from build123d import *

# Parameters (mm, degrees)
SKETCH2_R              = 26
BOSS_EXTRUDE2_DEPTH    = 5
SKETCH3_R              = 4
CUT_EXTRUDE1_DEPTH     = 2
CUT_EXTRUDE3_START     = -5
CUT_EXTRUDE3_OUTLINE_R = 26
CUT_EXTRUDE3_DEPTH     = 5


# Read off the part's stored shape, not the designer's step: Cut-Extrude3
with BuildPart() as part:
    # Sketch2 → Boss-Extrude2 (new body)
    with BuildSketch(Plane(origin=(0, 0, 0), x_dir=(1, 0, 0), z_dir=(0, 1, 0))):
        with Locations(Location((0, 0, 0), (0, 0, 270))):
            Circle(SKETCH2_R)
    extrude(amount=BOSS_EXTRUDE2_DEPTH)

    # Sketch3 → Cut-Extrude1 (cut)
    with BuildSketch(Plane.XZ.offset(-5)):
        with Locations(Location((9.52625, -16.499949006, 0), (0, 0, 270))):
            Circle(SKETCH3_R)
        with Locations(Location((9.52625, 16.499949006, 0), (0, 0, 270))):
            Circle(SKETCH3_R)
        with Locations(Location((-19.0525, 0, 0), (0, 0, 270))):
            Circle(SKETCH3_R)
    extrude(amount=CUT_EXTRUDE1_DEPTH, mode=Mode.SUBTRACT)

    # Cut-Extrude3 outline → Cut-Extrude3 (cut)
    # profile 1 of 2: a face of its own
    with BuildSketch(Plane(origin=(0, 5, 0), x_dir=(1, 0, 0), z_dir=(0, 1, 0)).offset(CUT_EXTRUDE3_START)):
        Circle(CUT_EXTRUDE3_OUTLINE_R)
        with BuildLine():
            ThreePointArc((-19.664092803, -5.96874813), (-25.0525, 0), (-19.664092803, 5.96874813))
            ThreePointArc((-19.664092803, 5.96874813), (-10.275, 17.796822048), (4.662958892, 20.013977975))
            ThreePointArc((4.662958892, 20.013977975), (12.52625, 21.696101428), (15.001133911, 14.045229844))
            ThreePointArc((15.001133911, 14.045229844), (20.55, 0), (15.001133911, -14.045229844))
            ThreePointArc((15.001133911, -14.045229844), (12.52625, -21.696101428), (4.662958892, -20.013977975))
            ThreePointArc((4.662958892, -20.013977975), (-10.275, -17.796822048), (-19.664092803, -5.96874813))
        make_face(mode=Mode.SUBTRACT)
    # profile 2 of 2: a face of its own
    with BuildSketch(Plane(origin=(0, 5, 0), x_dir=(1, 0, 0), z_dir=(0, 1, 0)).offset(CUT_EXTRUDE3_START)):
        with BuildLine():
            ThreePointArc((-16.664486452, 5.504306613), (-13.0525, 0), (-16.664486452, -5.504306613))
            ThreePointArc((-16.664486452, -5.504306613), (-8.775, -15.198745836), (3.565373869, -17.184021915))
            ThreePointArc((3.565373869, -17.184021915), (6.52625, -11.303796583), (13.099112583, -11.679715302))
            ThreePointArc((13.099112583, -11.679715302), (17.55, 0), (13.099112583, 11.679715302))
            ThreePointArc((13.099112583, 11.679715302), (6.52625, 11.303796583), (3.565373869, 17.184021915))
            ThreePointArc((3.565373869, 17.184021915), (-8.775, 15.198745836), (-16.664486452, 5.504306613))
        make_face()
    extrude(amount=CUT_EXTRUDE3_DEPTH, mode=Mode.SUBTRACT)


solid = part.part
Check sheet for the modelled part. Datum: model origin and axes. Units: mm. A direction names the side the tool comes from. Give positions to 0.01 mm unless a question says otherwise; leave off trailing zeros. Loops run counter-clockwise (first coordinate to the right, second up) from the corner with the lowest first, then second, coordinate; pieces in that order, holes last. Notation, with made-up numbers: M -13.75,-5 L -2.75,-5 A16 ccw -2.75,6 Z; hole C 76.5,-1.5 d6. An arc over 180 degrees is marked long. Answer as a JSON object with one key per item and string values. Group by question number.
Q1. Access from +Z, -Z, +X, -X, +Y, -Y to the whole of each face (thin tool, end or side, straight path). Record for faces 4 (the cylindrical face through (6.611, 2.465, -11.256)), 5 (the cylindrical face through (-25.05, 2.46, 0.12)), 6 (the flat face through (10, 3, 17)).
Q2. Go/stop test with flat-tipped pins: P1, Ø5, axis at x = 9.53, z = 16.5, coming from the -Y side; P2, Ø2, axis at x = -12, z = -0.5, coming from the +Y side; P3, Ø2, axis at x = -19, y = 3.5, coming from the -Z side; P4, Ø2, axis at x = 6.5, y = 3, coming from the -Z side. Record where each tip stops, or that it passes through.
Q3. Material ranges on line 1 along X through (y, z) = (4.65, 1.5); line 2 along X through (y, z) = (2.4, -11); line 3 along Z through (x, y) = (9, 4.2), recorded low to high. Write a range as [from, to].
Q4. Cross-section at C-C on x = 1.5. Record the cut outline in (y, z).
Q5. Cross-section at D-D on z = -6.5. Record the cut outline in (x, y), then the cut area to 3 significant figures.
Q6. Release check for a two-part mould opening along Z. For faces 1 (the flat face through (6, 5, -12)), 2 (the flat face through (10, 3, -16)), 3 (the cylindrical face through (-10.46, 2.46, -17.69)) record: released by +Z, released by -Z, zero draft, split by the parting line, or undercut.
Q7. Cross-section at A-A on z = 0. Record the cut outline in (x, y).
Q8. Cross-section at B-B on x = 7. Record the cut outline in (y, z).
Evaluation:
{
 "1": {"face 4": "+Y, -Y", "face 5": "-X, +Y, -Y", "face 6": "+Y"},
 "2": {"P1": "stops at y = 0", "P2": "passes through", "P3": "stops at z = -9.91", "P4": "stops at z = -22.15"},
 "3": {"line 1": "x = [-24.86, -22.76], [-15.34, -13.24], [17.49, 20.5]", "line 2": "x = [-17.36, -13.67], [7.13, 11.92], [13.67, 17.36]", "line 3": "z = [-22.48, -20.47], [-12.53, -10.52], [10.52, 12.53], [20.47, 22.48]"},
 "4": {"outline": "M 0,-20.5 L 5,-20.5 L 5,-17.49 L 0,-17.49 Z; M 0,17.49 L 5,17.49 L 5,20.5 L 0,20.5 Z"},
 "5": {"outline": "M -19.49,0 L -16.3,0 L -16.3,5 L -19.49,5 Z; M 16.3,0 L 19.49,0 L 19.49,5 L 16.3,5 Z", "area": "31.9 mm2"},
 "6": {"face 1": "zero draft", "face 2": "undercut", "face 3": "released by -Z"},
 "7": {"outline": "M -25.05,0 L -13.05,0 L -13.05,5 L -15.05,5 L -15.05,3 L -23.05,3 L -23.05,5 L -25.05,5 Z; M 17.55,0 L 20.55,0 L 20.55,5 L 17.55,5 Z"},
 "8": {"outline": "M 0,-21.94 L 5,-21.94 L 5,-19.6 L 3,-19.6 L 3,-13.4 L 5,-13.4 L 5,-11.06 L 0,-11.06 Z; M 0,11.06 L 5,11.06 L 5,13.4 L 3,13.4 L 3,19.6 L 5,19.6 L 5,21.94 L 0,21.94 Z"}
}
